from build123d import *

# Parameters (mm, degrees)
F1_DEPTH    = 50
F2_DEPTH    = 37.5
F4_T1_DEPTH = 103.3030187921
F4_T3_DEPTH = 91.394543157
F4_T5_DEPTH = 93.4430330881


# Not quite as in the source:
# - a fillet or chamfer that OpenCascade refuses, or shapes differently, is made with other operations: its cross-section is extruded or revolved along the edge and cut away or added


with BuildPart() as f1:
    # F0 (on Front) → F1 (new body, symmetric)
    with BuildSketch(Plane.XZ):
        with BuildLine():
            Line((-59.8632097244, -15.5979888514), (59.8632097244, -15.5979888514))
            ThreePointArc((59.8632097244, -15.5979888514), (75.4611985758, 0), (59.8632097244, 15.5979888514))
            Line((59.8632097244, 15.5979888514), (47.2922846675, 15.5979888514))
            Line((47.2922846675, 15.5979888514), (-46.2039783597, 15.5979888514))
            Line((-46.2039783597, 15.5979888514), (-59.8632097244, 15.5979888514))
            ThreePointArc((-59.8632097244, 15.5979888514), (-75.4611985758, 0), (-59.8632097244, -15.5979888514))
        make_face()
    extrude(amount=F1_DEPTH, both=True)

    # F0 (on Front) → F2 (join, symmetric)
    with BuildSketch(Plane.XZ):
        Polygon((-46.2039783597, 15.5979888514), (47.2922846675, 15.5979888514), (38.0605123937, 34.2928767204), (20.7754876465, 34.2928767204), (4.2761466466, 34.2928767204), (-12.2231943533, 34.2928767204), (-39.5256765187, 34.2928767204), align=None)
    extrude(amount=F2_DEPTH, both=True)

    # F0 (on Front) → F3 (revolve)
    with BuildSketch(Plane.XZ):
        with BuildLine():
            Line((4.2761466466, 34.2928767204), (20.7754876465, 34.2928767204))
            Line((20.7754876465, 34.2928767204), (20.7754876465, 42.9353863001))
            ThreePointArc((20.7754876465, 42.9353863001), (15.9429425527, 54.6021822062), (4.2761466466, 59.4347273))
            Line((4.2761466466, 59.4347273), (4.2761466466, 42.9353863001))
            Line((4.2761466466, 42.9353863001), (4.2761466466, 34.2928767204))
        make_face()
    revolve(axis=Axis((4.2761466466, 0, 51.1850568), (0, 0, 1)))

    # F4: chamfer of 5 on 4 edges, made by hand

    # F4_s2 → F4_t1 (cut)
    with BuildSketch(Plane.YZ.offset(-52.3840914585)):
        Polygon((-37.5, 29.2928767204), (-32.5, 34.2928767204), (-37.5, 34.2928767204), align=None)
        Polygon((37.5, 29.2928767204), (32.5, 34.2928767204), (37.5, 34.2928767204), align=None)
    extrude(amount=F4_T1_DEPTH, mode=Mode.SUBTRACT)

    # F4_s4 → F4_t3 (cut)
    with BuildSketch(Plane.XZ.offset(-45.6972715785)):
        Polygon((39.4363488807, 31.506726013), (34.9531724053, 34.2928767204), (38.0605123937, 34.2928767204), align=None)
    extrude(amount=F4_T3_DEPTH, mode=Mode.SUBTRACT)

    # F4_s6 → F4_t5 (cut)
    with BuildSketch(Plane.XZ.offset(-46.7215165441)):
        Polygon((-40.7109421413, 30.9749063085), (-36.0023567418, 34.2928767204), (-39.5256765187, 34.2928767204), align=None)
    extrude(amount=F4_T5_DEPTH, mode=Mode.SUBTRACT)


solid = f1.part
Could you check a few things on this model? Use its own coordinates, in mm. A direction names the side the tool comes from. Coordinates: 2 decimals unless noted, no trailing zeros. Order: outer loops, then holes, each group sorted by start corner. A loop starts at its lowest first (then second) coordinate and runs counter-clockwise, first axis right, second up.
Q1. Suppose I cut it at D-D on x = 42.5. Please give me the cut outline in (y, z).
Q2. Suppose I cut it at A-A on x = -14.5. Please give me the cut outline in (y, z).
Q3. Suppose I cut it at B-B on y = 23. Please give me the cut outline in (x, z).
Q4. Suppose I cut it at C-C on y = 0. Please give me the cut outline in (x, z), and give its area (3 significant figures).
Q5. Please list where these lines run through material, in increasing order: L1, parallel to Z at x = 48, y = 28.5; L2, parallel to Y at x = -7, z = 23; L3, parallel to Z at x = -9, y = 12.5.
Q6. Will these pins go through, and if not, where does the flat tip stop? pin 1 (1 mm diameter, centred on y = -5.5, z = 21, fed in from +X); pin 2 (6 mm diameter, centred on x = -29, y = 16.5, fed in from +Z); pin 3 (4 mm diameter, centred on x = -49.5, y = 10.5, fed in from +Z).
Q7. Which directions (+Z, -Z, +X, -X, +Y, -Y) give clear straight access to the entire face, cutting with the end or side of a thin tool? Please do faces 1 (the flat face through (37.23, 0.49, 32.88)), 2 (the cylindrical face through (0.699, -16.107, 38.675)), 3 (the flat face through (0, 37.5, 23)), 4 (the flat face through (0, -37.5, 23)).
Answer:
1. outline: (-50, -15.6) - (50, -15.6) - (50, 15.6) - (37.5, 15.6) - (37.5, 25.3) - (-37.5, 25.3) - (-37.5, 15.6) - (-50, 15.6) - close
2. outline: (-50, -15.6) - (50, -15.6) - (50, 15.6) - (37.5, 15.6) - (37.5, 29.29) - (32.5, 34.29) - (-32.5, 34.29) - (-37.5, 29.29) - (-37.5, 15.6) - (-50, 15.6) - close
3. outline: (-59.86, -15.6) - (59.86, -15.6) arc R15.6 ccw to (59.86, 15.6) - (47.29, 15.6) - (39.44, 31.51) - (34.95, 34.29) - (-36, 34.29) - (-40.71, 30.97) - (-46.2, 15.6) - (-59.86, 15.6) arc R15.6 ccw to start
4. outline: (-59.86, -15.6) - (59.86, -15.6) arc R15.6 ccw to (59.86, 15.6) - (47.29, 15.6) - (39.44, 31.51) - (34.95, 34.29) - (20.78, 34.29) - (20.78, 42.94) arc R16.5 ccw to (-12.22, 42.94) - (-12.22, 34.29) - (-36, 34.29) - (-40.71, 30.97) - (-46.2, 15.6) - (-59.86, 15.6) arc R15.6 ccw to start
4. area: 6,800 mm2
5. L1: z = -15.6 to 15.6
5. L2: y = -37.5 to 37.5
5. L3: z = -15.6 to 34.29
6. pin 1: stops at x = 44.87
6. pin 2: stops at z = 34.29
6. pin 3: stops at z = 15.6
7. face 1: +Z, +X, +Y, -Y
7. face 2: +Z
7. face 3: +Z, +X, -X, +Y
7. face 4: +Z, +X, -X, -Y
